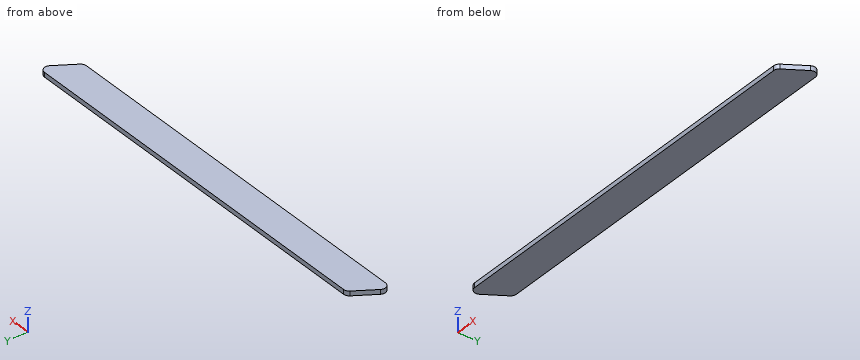
from build123d import *

# Parameters (mm, degrees)
SKETCH1_W           = 145
SKETCH1_H           = 11
BOSS_EXTRUDE1_DEPTH = 1.6
CUT_EXTRUDE1_DEPTH  = 73.725923851
FILLET2_R           = 2


with BuildPart() as part:
    # Sketch1 → Boss-Extrude1 (new body)
    with BuildSketch(Plane.XY):
        Rectangle(SKETCH1_W, SKETCH1_H)
    extrude(amount=BOSS_EXTRUDE1_DEPTH)

    # Sketch2 → Cut-Extrude1 (cut, through all)
    with BuildSketch(Plane.XY.offset(1.6)):
        Polygon((-72.5, -5.5), (-65.5, 5.5), (-72.5, 5.5), align=None)
        Polygon((72.5, 5.5), (65.5, -5.5), (72.5, -5.5), align=None)
    extrude(amount=-CUT_EXTRUDE1_DEPTH, mode=Mode.SUBTRACT)

    # Fillet2
    fillet2_edges = [part.edges().sort_by_distance(p)[0] for p in [
        (-65.5, 5.5, 0.8),
        (65.5, -5.5, 0.8),
        (-72.5, -5.5, 0.8),
        (72.5, 5.5, 0.8),
    ]]
    fillet(fillet2_edges, radius=FILLET2_R)


solid = part.part
The listing builds one solid part. Answer for the finished solid, in the listing's coordinates (mm). Coordinates: 2 decimals unless noted, no trailing zeros. Write each loop counter-clockwise with the first axis right and the second up, starting at its lowest first coordinate (ties: lowest second). Pieces come first, ordered by that corner, then holes. Notation, with made-up numbers: M 32,-14 L 53,-14 A23 cw 53,9 Z; hole C -13,-24.5 d4. An arc over 180 degrees is marked long. Put each result on its own line as item: value. Start each with the question number.
1. A cutting plane is placed at A-A on z = 0.25. Write down the section's boundary in (x, y).
2. A cutting plane is placed at B-B on y = 0. Write down the section's boundary in (x, z), then the cut area to 3 significant figures.
3. Consider line 1 (X direction, y = 4.75, z = 0.55); line 2 (X direction, y = 0, z = 0.7). Determine where each line is inside the solid, lowest interval first. Write a range as from..to.
Resolved:
1. outline: M -70.54,-2.43 A2 ccw -68.86,-5.5 L 64.4,-5.5 A2 ccw 66.09,-4.57 L 70.54,2.43 A2 ccw 68.86,5.5 L -64.4,5.5 A2 ccw -66.09,4.57 Z
2. outline: M -69,0 L 69,0 L 69,1.6 L -69,1.6 Z
2. area: 221 mm2
3. line 1: x = -65.96..70.42
3. line 2: x = -69..69
